```python
from build123d import *

# Parameters (mm, degrees)
OBJ1_R           = 13.0683
OBJ1_DEPTH       = 51.7525
OBJ1_ROLL_ANGLE  = -90
OBJ2_R           = 13.0683
OBJ2_DEPTH       = 51.7525
OBJ3_R                = 16.7767
OBJ3_DEPTH            = 31.7754
OBJ3_PITCH_ANGLE      = 90
OBJ4_R                = 16.7767
OBJ4_DEPTH            = 31.7754
OBJ4_ROLL_ANGLE       = -90
OBJ5_R                = 16.7767
OBJ5_DEPTH            = 31.7754
OBJ6           = 13.0683
OBJ7       = 51.7525
OBJ8 = 90
OBJ9_R              = 20.2565
OBJ9_DEPTH          = 51.7525
OBJ9_ROLL_ANGLE     = -90
OBJ10_R              = 20.2565
OBJ10_DEPTH          = 51.7525
OBJ11              = 20.2565
OBJ12          = 51.7525
OBJ13    = 90


with BuildPart() as obj1:
    # obj1 → obj1 (new body)
    with BuildSketch(Plane.XY):
        Circle(OBJ1_R)
    extrude(amount=OBJ1_DEPTH)


with BuildPart() as obj1_1:
    # obj1 roll: moved
    add(obj1.part.rotate(Axis((0, 0, 0), (1, 0, 0)), OBJ1_ROLL_ANGLE))


with BuildPart() as obj1_2:
    # obj1 placement: moved
    add(obj1_1.part)


with BuildPart() as obj2:
    # obj2 → obj2 (new body)
    with BuildSketch(Plane.XY):
        Circle(OBJ2_R)
    extrude(amount=OBJ2_DEPTH)


with BuildPart() as sphere001:
    # Sphere001 → Sphere001 (revolve)
    with BuildSketch(Plane.XZ):
        with BuildLine():
            ThreePointArc((0, -13.0683), (13.0683, 0), (0, 13.0683))
            Line((0, 13.0683), (0, -13.0683))
        make_face()
    revolve(axis=Axis((0, 0, 0), (0, 0, 1)))


with BuildPart() as obj3:
    # obj3 → obj3 (new body)
    with BuildSketch(Plane.XY):
        Circle(OBJ3_R)
    extrude(amount=OBJ3_DEPTH)


with BuildPart() as obj3_1:
    # obj3 pitch: moved
    add(obj3.part.rotate(Axis((0, 0, 0), (0, 1, 0)), OBJ3_PITCH_ANGLE))


with BuildPart() as obj3_2:
    # obj3 placement: moved
    add(obj3_1.part.moved(Location((19.9771, 0, 0))))


with BuildPart() as obj4:
    # obj4 → obj4 (new body)
    with BuildSketch(Plane.XY):
        Circle(OBJ4_R)
    extrude(amount=OBJ4_DEPTH)


with BuildPart() as obj4_1:
    # obj4 roll: moved
    add(obj4.part.rotate(Axis((0, 0, 0), (1, 0, 0)), OBJ4_ROLL_ANGLE))


with BuildPart() as obj4_2:
    # obj4 placement: moved
    add(obj4_1.part.moved(Location((0, 19.9771, 0))))


with BuildPart() as obj5:
    # obj5 → obj5 (new body)
    with BuildSketch(Plane.XY.offset(19.9771)):
        Circle(OBJ5_R)
    extrude(amount=OBJ5_DEPTH)


with BuildPart() as fusion001:
    with BuildSketch(Plane.XY):
        Circle(OBJ6)
    extrude(amount=OBJ7)


with BuildPart() as fusion001_1:
    add(fusion001.part.rotate(Axis((0, 0, 0), (0, 1, 0)), OBJ8))


with BuildPart() as fusion001_2:
    add(fusion001_1.part)

    # Fusion001: union obj1, obj2, Sphere001, obj3, obj4, obj5
    add(obj1_2.part)
    add(obj2.part)
    add(sphere001.part)
    add(obj3_2.part)
    add(obj4_2.part)
    add(obj5.part)


with BuildPart() as obj9:
    # obj9 → obj9 (new body)
    with BuildSketch(Plane.XY):
        Circle(OBJ9_R)
    extrude(amount=OBJ9_DEPTH)


with BuildPart() as obj9_1:
    # obj9 roll: moved
    add(obj9.part.rotate(Axis((0, 0, 0), (1, 0, 0)), OBJ9_ROLL_ANGLE))


with BuildPart() as obj9_2:
    # obj9 placement: moved
    add(obj9_1.part)


with BuildPart() as obj10:
    # obj10 → obj10 (new body)
    with BuildSketch(Plane.XY):
        Circle(OBJ10_R)
    extrude(amount=OBJ10_DEPTH)


with BuildPart() as sphere:
    # Sphere → Sphere (revolve)
    with BuildSketch(Plane.XZ):
        with BuildLine():
            ThreePointArc((0, -20.2565), (20.2565, 0), (0, 20.2565))
            Line((0, 20.2565), (0, -20.2565))
        make_face()
    revolve(axis=Axis((0, 0, 0), (0, 0, 1)))


with BuildPart() as f0013we:
    with BuildSketch(Plane.XY):
        Circle(OBJ11)
    extrude(amount=OBJ12)


with BuildPart() as f0013we_1:
    add(f0013we.part.rotate(Axis((0, 0, 0), (0, 1, 0)), OBJ13))


with BuildPart() as f0013we_2:
    add(f0013we_1.part)

    # Fusion: union obj9, obj10, Sphere
    add(obj9_2.part)
    add(obj10.part)
    add(sphere.part)

    # Cut: cut Fusion001
    add(fusion001_2.part, mode=Mode.SUBTRACT)


solid = f0013we_2.part
```
Here's how the part is built. I have some questions about the finished solid (model axes, mm). A direction names the side the tool comes from. Give positions to 0.01 mm unless a question says otherwise; leave off trailing zeros. Order: outer loops, then holes, each group sorted by start corner. A loop starts at its lowest first (then second) coordinate and runs counter-clockwise, first axis right, second up. Notation, with made-up numbers: (-26.75, 69.25) - (28.25, 69.25) arc R15 cw to (28.25, 81.25) - close; hole circle Ø7 at (65.5, 82.5). An arc over 180 degrees is marked (long way). Answer as a JSON object with one key per item and string values. Group by question number.
Item 1: For P1, Ø6, axis at x = 44, y = 10.5, coming from the -Z side; P2, Ø1.5, axis at x = 31, y = -2, coming from the +Z side; P3, Ø3, axis at y = -12.5, z = 36, coming from the -X side; P4, Ø2, axis at x = 27, y = -0.5, coming from the -Z side, each with a flat end and sliding along its axis, tell me the tip position at first contact or that it passes through.
Item 2: If we section it at D-D on x = -14.5: Please give me the cut outline in (y, z), and give its area (3 significant figures).
Item 3: If we section it at A-A on y = 22.5: Please give me the cut outline in (x, z).
Item 4: If we mould it in two halves opening along Y, with no side actions, what happens to faces 5 (the flat face through (9, 19.977, 10)), 6 (the flat face through (51.752, 15, 8)), 7 (the flat face through (9, -10, 19.977))? For each: pulls with the +Y half, pulls with the -Y half, needs draft (parallel to the pull), parting line crosses it, or undercut.
Item 5: If we section it at B-B on y = 6.5: Please give me the cut outline in (x, z).
Item 6: Please list where these lines run through material, in increasing order: probe 1 along Z at (x, y) = (0, 41); probe 2 along Y at (x, z) = (0, 5).
Item 7: Which directions (+Z, -Z, +X, -X, +Y, -Y) give clear straight access to the entire face, cutting with the end or side of a thin tool? Please do faces 1 (the flat face through (-8, 51.752, -15)), 2 (the cylindrical face through (-9.632, 12.068, -8.832)), 3 (the flat face through (19.977, -10, -9)), 4 (the cylindrical face through (-10.37, -7.95, 12.07)).
Result set:
{
 "1": {"P1": "z = -18.82", "P2": "z = 20.22", "P3": "x = -17.01", "P4": "z = -20.26"},
 "2": {"outline": "(-14.14, 0) arc R14.14 ccw to (0, -14.14) - (51.75, -14.14) - (51.75, -8.44) - (19.98, -8.44) - (19.98, 8.44) - (51.75, 8.44) - (51.75, 14.14) - (14.14, 14.14) - (14.14, 51.75) - (8.44, 51.75) - (8.44, 19.98) - (-8.44, 19.98) - (-8.44, 51.75) - (-14.14, 51.75) - close", "area": "1,810 mm²"},
 "3": {"outline": "circle Ø40.51 at (0, 0); hole circle Ø33.55 at (0, 0)"},
 "4": {"face 5": "pulls with the +Y half", "face 6": "needs draft", "face 7": "undercut"},
 "5": {"outline": "(-19.19, 6.5) arc R20.26 ccw to (6.5, -19.19) - (51.75, -19.19) - (51.75, -15.47) - (19.98, -15.47) - (19.98, -11.34) - (6.5, -11.34) arc R13.07 cw to (-11.34, 6.5) - (-11.34, 19.98) - (-15.47, 19.98) - (-15.47, 51.75) - (-19.19, 51.75) - close; (11.34, 11.34) - (19.98, 11.34) - (19.98, 15.47) - (51.75, 15.47) - (51.75, 19.19) - (19.19, 19.19) - (19.19, 51.75) - (15.47, 51.75) - (15.47, 19.98) - (11.34, 19.98) - close"},
 "6": {"probe 1": "-20.26 to -16.78, 16.78 to 20.26", "probe 2": "-20.26 to -13.07"},
 "7": {"face 1": "+Z, -Z, +X, -X, +Y", "face 2": "+Y", "face 3": "+X", "face 4": "+Z"}
}
